```python
from build123d import *

# Parameters (mm, degrees)
SKETCH_1_W      = 116
SKETCH_1_H      = 116
EXTRUDE_1_DEPTH = 20
SHELL_1_T       = -3
SKETCH_2_W      = 122
SKETCH_2_H      = 122
EXTRUDE_2_DEPTH = 5
SKETCH_4_W      = 30
SKETCH_4_H      = 30
SKETCH_4_W_2    = 26
SKETCH_4_H_2    = 26
EXTRUDE_3_DEPTH = 165


with BuildPart() as part:
    # 草图1 → 凸台-拉伸1 (new body)
    with BuildSketch(Plane(origin=(0, 0, 0), x_dir=(1, 0, 0), z_dir=(0, 1, 0))):
        Rectangle(SKETCH_1_W, SKETCH_1_H)
    extrude(amount=EXTRUDE_1_DEPTH)

    # 抽壳1
    shell_1_openings = [part.faces().sort_by_distance(p)[0] for p in [
        (0, 20, 0),
    ]]
    offset(amount=SHELL_1_T, openings=shell_1_openings, kind=Kind.INTERSECTION)

    # 草图2 → 凸台-拉伸2 (add)
    with BuildSketch(Plane.XZ):
        Rectangle(SKETCH_2_W, SKETCH_2_H)
    extrude(amount=EXTRUDE_2_DEPTH)

    # 草图4 → 凸台-拉伸3 (add)
    with BuildSketch(Plane.XZ.offset(5)):
        with Locations((-31, 31)):
            Rectangle(SKETCH_4_W, SKETCH_4_H)
        with Locations((-31, 31)):
            Rectangle(SKETCH_4_W_2, SKETCH_4_H_2, mode=Mode.SUBTRACT)
    extrude(amount=EXTRUDE_3_DEPTH)


solid = part.part
```
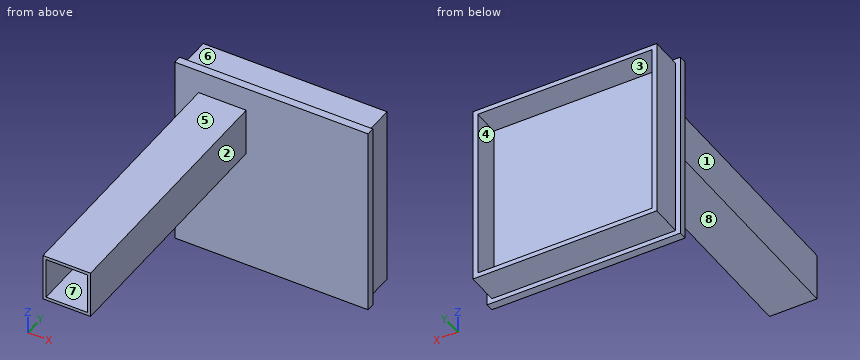
Input: part model. Units: mm. Frame: model coordinates. Face numbers are marked on the shaded views. A direction names the side the tool comes from. Give positions to 0.01 mm unless a question says otherwise; leave off trailing zeros. Order: outer loops, then holes, each group sorted by start corner. A loop starts at its lowest first (then second) coordinate and runs counter-clockwise, first axis right, second up. Notation, with made-up numbers: (38.25, -15) -> (63.25, -15) arc R19 ccw to (63.25, 8) -> close; hole circle Ø5 at (0.5, 57). An arc over 180 degrees is marked (long way). Write each question's results on one line, items separated by ' | '. Start each with the question number.
Item 1: Line query: line 1 (Z direction, x = -23.5, y = -19); line 2 (X direction, y = -57, z = 27); line 3 (Y direction, x = 46, z = -2). Output: solid intervals per line, ascending.
Item 2: Cut plane D-D on z = -10.5. Return the cut outline in (x, y), then the cut area to 3 significant figures.
Item 3: Mould query, pull axis X, two halves, no side actions, for the marked faces 1, 2 and 3. Classes: pulls with the +X half, pulls with the -X half, needs draft (parallel to the pull), parting line crosses it, or undercut.
Item 4: Set-up query: the marked faces 4, 5, 6, 7 and 8. Return all of +Z, -Z, +X, -X, +Y, -Y with unobstructed straight access to the full face (end or side cutting, diameter ignored); none if empty.
Item 5: Cut plane B-B on y = -66. Return the cut outline in (x, z), then the cut area to 3 significant figures.
Item 6: Cut plane C-C on x = -29. Return the cut outline in (y, z).
Item 7: Contact query for flat-ended pins moving along their axis: P1, Ø22, axis at x = -3.5, y = 12, coming from the +Z side; P2, Ø3, axis at x = -44.5, z = 6.5, coming from the -Y side; P3, Ø12, axis at y = -22, z = 11.5, coming from the -X side; P4, Ø3, axis at y = -9.5, z = 14, coming from the -X side. Output: stop coordinate, or through.
Item 8: Cut plane A-A on z = 25. Return the cut outline in (x, y).
Established:
1) line 1: 16 to 18, 44 to 46 | line 2: -46 to -44, -18 to -16 | line 3: -5 to 3
2) outline: (-61, -5) -> (61, -5) -> (61, 0) -> (58, 0) -> (58, 20) -> (55, 20) -> (55, 3) -> (-55, 3) -> (-55, 20) -> (-58, 20) -> (-58, 0) -> (-61, 0) -> close | area: 1,060 mm^2
3) face 1: pulls with the -X half | face 2: pulls with the +X half | face 3: undercut
4) face 4: +Y | face 5: +Z, +X, -X, -Y | face 6: +Z, +X, -X, +Y | face 7: -Y | face 8: -Z, +X, -X, -Y
5) outline: (-46, 16) -> (-16, 16) -> (-16, 46) -> (-46, 46) -> close; hole (-44, 18) -> (-18, 18) -> (-18, 44) -> (-44, 44) -> close | area: 224 mm^2
6) outline: (-170, 16) -> (-5, 16) -> (-5, -61) -> (0, -61) -> (0, -58) -> (20, -58) -> (20, -55) -> (3, -55) -> (3, 55) -> (20, 55) -> (20, 58) -> (0, 58) -> (0, 61) -> (-5, 61) -> (-5, 46) -> (-170, 46) -> (-170, 44) -> (-5, 44) -> (-5, 18) -> (-170, 18) -> close
7) P1: z = 58 | P2: y = -5 | P3: x = -46 | P4: through
8) outline: (-61, -5) -> (-46, -5) -> (-46, -170) -> (-44, -170) -> (-44, -5) -> (-18, -5) -> (-18, -170) -> (-16, -170) -> (-16, -5) -> (61, -5) -> (61, 0) -> (58, 0) -> (58, 20) -> (55, 20) -> (55, 3) -> (-55, 3) -> (-55, 20) -> (-58, 20) -> (-58, 0) -> (-61, 0) -> close
